Input: part model. Units: mm. Frame: model coordinates. Round coordinates to 2 decimals unless told otherwise and drop trailing zeros. Loops run counter-clockwise (first coordinate to the right, second up) from the corner with the lowest first, then second, coordinate; pieces in that order, holes last. Notation, with made-up numbers: (23.5, -33.75) -> (64.5, -33.75) arc R23 cw to (64.5, -25.75) -> close; hole circle Ø11 at (-2.75, -22.5). An arc over 180 degrees is marked (long way). One line per question, with ' | ' between items. Start each with the question number.
Q1. Contact query for flat-ended pins moving along their axis: P1, Ø3, axis at y = 3.5, z = 46.5, coming from the -X side; P2, Ø1.7, axis at x = 0, y = 0, coming from the -Z side; P3, Ø1, axis at x = 0.5, z = 7, coming from the +Y side. Output: stop coordinate, or through.
Q2. Material intervals for L1, parallel to X at y = 0, z = 34.5; L2, parallel to Y at x = 0, z = 47, sorted ascending.
Q3. Cut plane C-C on z = 19.5. Return loops of the section in (x, y), and give its area (3 significant figures).
Q4. Cut plane A-A on x = 0. State how many separate pieces and enclosed holes the cut face has, and give its area (3 significant figures).
Q5. Cut plane D-D on y = 6. Return loops of the section in (x, z), and give its area (3 significant figures).
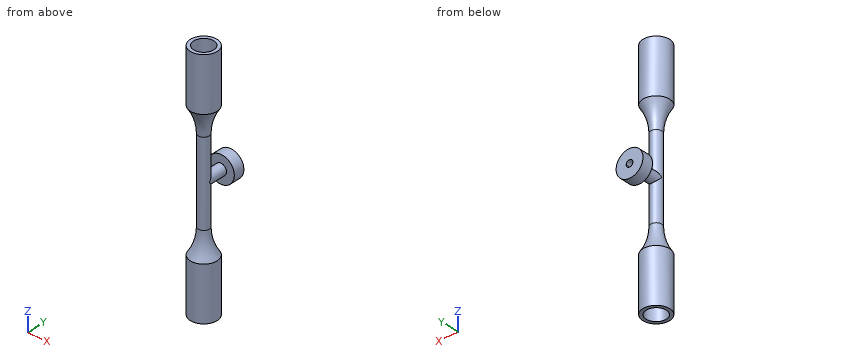
from build123d import *

# Parameters (mm, degrees)
SKETCH1_R           = 3
BOSS_EXTRUDE1_DEPTH = 12
SKETCH2_R           = 1.25
BOSS_EXTRUDE2_DEPTH = 15
BOSS_EXTRUDE3_DEPTH = 4.5
BOSS_EXTRUDE4_DEPTH = 2.5
SKETCH5_R           = 2.25
CUT_EXTRUDE1_DEPTH  = 10.5
SKETCH6_R           = 0.75
CUT_EXTRUDE2_DEPTH  = 21.5
CUT_EXTRUDE3_DEPTH  = 7
FILLET1_R           = 10


with BuildPart() as part:
    # Sketch1 → Boss-Extrude1 (new body)
    with BuildSketch(Plane.XY):
        Circle(SKETCH1_R)
    extrude(amount=BOSS_EXTRUDE1_DEPTH)

    # Sketch2 → Boss-Extrude2 (add)
    with BuildSketch(Plane.XY.offset(12)):
        Circle(SKETCH2_R)
    extrude(amount=BOSS_EXTRUDE2_DEPTH)

    # Sketch3 → Boss-Extrude3 (add)
    with BuildSketch(Plane(origin=(0, 0, 0), x_dir=(1, 0, 0), z_dir=(0, 1, 0))):
        with BuildLine():
            Line((-1.25, -27), (1.25, -27))
            ThreePointArc((1.25, -27), (0, -25.75), (-1.25, -27))
        make_face()
    extrude(amount=BOSS_EXTRUDE3_DEPTH)

    # Sketch4 → Boss-Extrude4 (add)
    with BuildSketch(Plane(origin=(0, 4.5, 0), x_dir=(1, 0, 0), z_dir=(0, 1, 0))):
        with BuildLine():
            Line((-3, -27), (3, -27))
            ThreePointArc((3, -27), (0, -24), (-3, -27))
        make_face()
    extrude(amount=BOSS_EXTRUDE4_DEPTH)

    # Sketch5 → Cut-Extrude1 (cut)
    with BuildSketch(Plane(origin=(0, 0, 0), x_dir=(-1, 0, 0), z_dir=(0, 0, -1))):
        Circle(SKETCH5_R)
    extrude(amount=-CUT_EXTRUDE1_DEPTH, mode=Mode.SUBTRACT)

    # Sketch6 → Cut-Extrude2 (cut)
    with BuildSketch(Plane.XY.offset(27)):
        Circle(SKETCH6_R)
    extrude(amount=-CUT_EXTRUDE2_DEPTH, mode=Mode.SUBTRACT)

    # Sketch7 → Cut-Extrude3 (cut)
    with BuildSketch(Plane(origin=(0, 7, 0), x_dir=(1, 0, 0), z_dir=(0, 1, 0))):
        with BuildLine():
            Line((-0.75, -27), (-0.75, -27.055459171))
            Line((-0.75, -27.055459171), (0.75, -27.055459171))
            Line((0.75, -27.055459171), (0.75, -27))
            ThreePointArc((0.75, -27), (0, -26.25), (-0.75, -27))
        make_face()
    extrude(amount=-CUT_EXTRUDE3_DEPTH, mode=Mode.SUBTRACT)

    # Fillet1
    # the kernel refuses this fillet: 10 mm, written as the material it adds along each edge
    with BuildSketch(Plane(origin=(0, 0, 12), x_dir=(1, 0, 0), z_dir=(0, -1, 0))) as fillet1_piece_1:
        with BuildLine():
            CenterArc((11.25, 5.651327278), FILLET1_R, 180, 34.41150867)
            Line((3, 0), (2.835, -0.113026546))
            ThreePointArc((2.835, -0.113026546), (2.125, -0.2), (1.25, -0.2))
            Line((1.25, -0.2), (1.05, 0))
            Line((1.05, 0), (1.05, 5.651327278))
            Line((1.05, 5.651327278), (1.25, 5.651327278))
        make_face()
    revolve(axis=Axis((0, 0, 12), (0, 0, 1)))

    # Mirror5: part across plane


with BuildPart() as part_1:
    add(part.part)
    add(part.part.mirror(Plane.XY.offset(27)))


solid = part_1.part
Results:
1) P1: x = -2.24 | P2: z = 10.5 | P3: y = 3
2) L1: -1.25 to -0.75, 0.75 to 1.25 | L2: -3 to -2.25, 2.25 to 3
3) outline: circle Ø2.5 at (0, 0); hole circle Ø1.5 at (0, 0) | area: 3.14 mm^2
4) separate pieces: 3 | enclosed holes: 0 | area: 101 mm^2
5) outline: circle Ø6 at (0, 27); hole circle Ø1.5 at (0, 27) | area: 26.5 mm^2
